Verification items for the finished model (mm, model axes). Face numbers are marked on the shaded views. A direction names the side the tool comes from. Coordinates: 2 decimals unless noted, no trailing zeros. Write each loop counter-clockwise with the first axis right and the second up, starting at its lowest first coordinate (ties: lowest second). Pieces come first, ordered by that corner, then holes. Notation, with made-up numbers: (27, -22.5) -> (52, -22.5) arc R19 cw to (52, 11.5) -> close; hole circle Ø11 at (-7.75, 77.25). An arc over 180 degrees is marked (long way). Use a Markdown table: item, result. Add a question column.
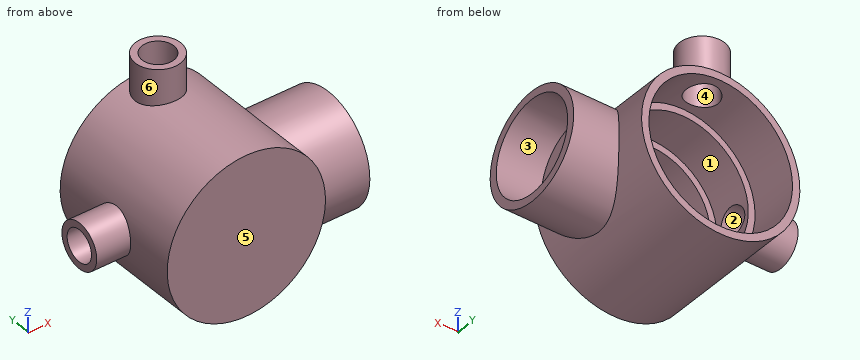
from build123d import *

# Parameters (mm, degrees)
SKETCH1_R                  = 35
BASE_DEPTH                 = 4
SKETCH2_R                  = 7.5
CENTERING_BOSS_DEPTH       = 2
SKETCH3_R                  = 35
SKETCH3_R_2                = 25.75
INLET_TIER_DEPTH           = 18
SKETCH4_R                  = 35
SKETCH4_R_2                = 28.75
PATIENT_TIER_DEPTH         = 18
SKETCH5_R                  = 35
SKETCH5_R_2                = 31.75
OUTLET_TIER_DEPTH          = 21.5
INLET_REACH                = 116.487
INLET_END_RADIUS           = 35
SKETCH7_R                  = 24
SKETCH10_R                 = 20.5
INLET_ID_DEPTH             = 20
INLET_PASS_THRU_REACH      = 101.535
INLET_PASS_THRU_END_RADIUS = 25.75
SKETCH11_R                 = 6
BOSS_EXTRUDE8_REACH        = 128.619
BOSS_EXTRUDE8_END_RADIUS   = 35
SKETCH12_R                 = 10
CUT_EXTRUDE3_REACH         = 128.619
CUT_EXTRUDE3_END_RADIUS    = 28.75
SKETCH13_R                 = 7
BOSS_EXTRUDE9_REACH        = 120.458
BOSS_EXTRUDE9_END_RADIUS   = 35
SKETCH14_R                 = 10
CUT_EXTRUDE4_REACH         = 120.458
CUT_EXTRUDE4_END_RADIUS    = 31.75
SKETCH15_R                 = 7


with BuildPart() as part:
    # Sketch1 → Base (new body)
    with BuildSketch(Plane(origin=(0, 0, 0), x_dir=(1, 0, 0), z_dir=(0, 1, 0))):
        with Locations(Location((0, 0, 0), (0, 0, 270))):
            Circle(SKETCH1_R)
    extrude(amount=BASE_DEPTH)

    # Sketch2 → Centering boss (add)
    with BuildSketch(Plane(origin=(0, 4, 0), x_dir=(1, 0, 0), z_dir=(0, 1, 0))):
        with Locations(Location((0, 0, 0), (0, 0, 270))):
            Circle(SKETCH2_R)
    extrude(amount=CENTERING_BOSS_DEPTH)

    # Sketch3 → Inlet tier (add)
    with BuildSketch(Plane(origin=(0, 4, 0), x_dir=(1, 0, 0), z_dir=(0, 1, 0))):
        with Locations(Location((0, 0, 0), (0, 0, 270))):
            Circle(SKETCH3_R)
        with Locations(Location((0, 0, 0), (0, 0, 270))):
            Circle(SKETCH3_R_2, mode=Mode.SUBTRACT)
    extrude(amount=INLET_TIER_DEPTH)

    # Sketch4 → Patient tier (add)
    with BuildSketch(Plane(origin=(0, 22, 0), x_dir=(1, 0, 0), z_dir=(0, 1, 0))):
        with Locations(Location((0, 0, 0), (0, 0, 270))):
            Circle(SKETCH4_R)
        with Locations(Location((0, 0, 0), (0, 0, 270))):
            Circle(SKETCH4_R_2, mode=Mode.SUBTRACT)
    extrude(amount=PATIENT_TIER_DEPTH)

    # Sketch5 → Outlet tier (add)
    with BuildSketch(Plane(origin=(0, 40, 0), x_dir=(1, 0, 0), z_dir=(0, 1, 0))):
        with Locations(Location((0, 0, 0), (0, 0, 270))):
            Circle(SKETCH5_R)
        with Locations(Location((0, 0, 0), (0, 0, 270))):
            Circle(SKETCH5_R_2, mode=Mode.SUBTRACT)
    extrude(amount=OUTLET_TIER_DEPTH)

    # Inlet: up to this cylinder (the profile starts outside it)
    inlet_end = Plane(origin=(0, 24.5, 0), z_dir=(0, -1, 0)) * Cylinder(INLET_END_RADIUS, 303.974, mode=Mode.PRIVATE)
    # Sketch7 → Inlet (add, up to the surface)
    with BuildSketch(Plane(origin=(55, 0, 0), x_dir=(0, 0, -1), z_dir=(1, 0, 0)), mode=Mode.PRIVATE) as inlet_sk1:
        with Locations((0, 24.5)):
            Circle(SKETCH7_R)
    inlet_tool1 = extrude(inlet_sk1.sketch, amount=-INLET_REACH, mode=Mode.PRIVATE) - inlet_end
    add(inlet_tool1.solids().sort_by_distance((55, 24.5, 0))[0])

    # Sketch10 → Inlet ID (cut)
    with BuildSketch(Plane(origin=(55, 0, 0), x_dir=(0, 0, -1), z_dir=(1, 0, 0))):
        with Locations((0, 24.5)):
            Circle(SKETCH10_R)
    extrude(amount=-INLET_ID_DEPTH, mode=Mode.SUBTRACT)

    # Inlet pass thru: up to this cylinder (the profile starts outside it)
    inlet_pass_thru_end = Plane(origin=(0, 14, 0), z_dir=(0, -1, 0)) * Cylinder(INLET_PASS_THRU_END_RADIUS, 255.57, mode=Mode.PRIVATE)
    # Sketch11 → Inlet pass thru (cut, up to the surface)
    with BuildSketch(Plane(origin=(35, 0, 0), x_dir=(0, 0, -1), z_dir=(1, 0, 0)), mode=Mode.PRIVATE) as inlet_pass_thru_sk1:
        with Locations((0, 14)):
            Circle(SKETCH11_R)
    inlet_pass_thru_tool1 = extrude(inlet_pass_thru_sk1.sketch, amount=-INLET_PASS_THRU_REACH, mode=Mode.PRIVATE) - inlet_pass_thru_end
    add(inlet_pass_thru_tool1.solids().sort_by_distance((35, 14, 0))[0], mode=Mode.SUBTRACT)

    # Boss-Extrude8: up to this cylinder (the profile starts outside it)
    boss_extrude8_end = Plane(origin=(0, 31, 0), z_dir=(0, -1, 0)) * Cylinder(BOSS_EXTRUDE8_END_RADIUS, 328.238, mode=Mode.PRIVATE)
    # Sketch12 → Boss-Extrude8 (add, up to the surface)
    with BuildSketch(Plane(origin=(-50, 0, 0), x_dir=(0, 0, -1), z_dir=(1, 0, 0)), mode=Mode.PRIVATE) as boss_extrude8_sk1:
        with Locations(Location((0, 31, 0), (0, 0, 180))):
            Circle(SKETCH12_R)
    boss_extrude8_tool1 = extrude(boss_extrude8_sk1.sketch, amount=BOSS_EXTRUDE8_REACH, mode=Mode.PRIVATE) - boss_extrude8_end
    add(boss_extrude8_tool1.solids().sort_by_distance((-50, 31, 0))[0])

    # Cut-Extrude3: up to this cylinder (the profile starts outside it)
    cut_extrude3_end = Plane(origin=(0, 31, 0), z_dir=(0, -1, 0)) * Cylinder(CUT_EXTRUDE3_END_RADIUS, 315.738, mode=Mode.PRIVATE)
    # Sketch13 → Cut-Extrude3 (cut, up to the surface)
    with BuildSketch(Plane.ZY.offset(50), mode=Mode.PRIVATE) as cut_extrude3_sk1:
        with Locations((0, 31)):
            Circle(SKETCH13_R)
    cut_extrude3_tool1 = extrude(cut_extrude3_sk1.sketch, amount=-CUT_EXTRUDE3_REACH, mode=Mode.PRIVATE) - cut_extrude3_end
    add(cut_extrude3_tool1.solids().sort_by_distance((-50, 31, 0))[0], mode=Mode.SUBTRACT)

    # Boss-Extrude9: up to this cylinder (the profile starts outside it)
    boss_extrude9_end = Plane(origin=(0, 50.75, 0), z_dir=(0, -1, 0)) * Cylinder(BOSS_EXTRUDE9_END_RADIUS, 311.916, mode=Mode.PRIVATE)
    # Sketch14 → Boss-Extrude9 (add, up to the surface)
    with BuildSketch(Plane.XY.offset(50), mode=Mode.PRIVATE) as boss_extrude9_sk1:
        with Locations((0, 50.75)):
            Circle(SKETCH14_R)
    boss_extrude9_tool1 = extrude(boss_extrude9_sk1.sketch, amount=-BOSS_EXTRUDE9_REACH, mode=Mode.PRIVATE) - boss_extrude9_end
    add(boss_extrude9_tool1.solids().sort_by_distance((0, 50.75, 50))[0])

    # Cut-Extrude4: up to this cylinder (the profile starts outside it)
    cut_extrude4_end = Plane(origin=(0, 50.75, 0), z_dir=(0, -1, 0)) * Cylinder(CUT_EXTRUDE4_END_RADIUS, 305.416, mode=Mode.PRIVATE)
    # Sketch15 → Cut-Extrude4 (cut, up to the surface)
    with BuildSketch(Plane.XY.offset(50), mode=Mode.PRIVATE) as cut_extrude4_sk1:
        with Locations((0, 50.75)):
            Circle(SKETCH15_R)
    cut_extrude4_tool1 = extrude(cut_extrude4_sk1.sketch, amount=-CUT_EXTRUDE4_REACH, mode=Mode.PRIVATE) - cut_extrude4_end
    add(cut_extrude4_tool1.solids().sort_by_distance((0, 50.75, 50))[0], mode=Mode.SUBTRACT)


solid = part.part
1) Release check for a two-part mould opening along X. For the marked faces 4, 5 and 6 record: released by +X, released by -X, zero draft, split by the parting line, or undercut.
2) Thickness scan on L1, parallel to Y at x = 0, z = 38.75; L2, parallel to Y at x = 40, z = 0; L3, parallel to Z at x = -41, y = 31. Record the ranges inside material, lowest first.
3) Cross-section at A-A on x = 0. Record the boundary of the cut face in (y, z), then the cut area to 3 significant figures.
4) Cross-section at D-D on y = 14. Record the boundary of the cut face in (x, z).
5) Cross-section at B-B on z = -18. Record the boundary of the cut face in (x, y).
6) Cross-section at C-C on x = -20. Record the boundary of the cut face in (y, z), then the cut area to 3 significant figures.
7) Set-up check for the marked faces 1, 2 and 3: record each of +Z, -Z, +X, -X, +Y, -Y from which the full face is reachable in a straight line by a thin tool's end or side.
8) Gauge pin test, flat ends, axial feed: pin 1 (19 mm diameter, centred on y = 14, z = 0, fed in from -X); pin 2 (20.5 mm diameter, centred on y = 19, z = 2.5, fed in from +X); pin 3 (1 mm diameter, centred on y = 13.5, z = -21.5, fed in from -X); pin 4 (2 mm diameter, centred on y = 10.5, z = -7.5, fed in from -X). Record the tip position at first contact, or that the pin passes through.
Returned:
| question | item | result |
|---|---|---|
| 1 | face 4 | undercut |
| 1 | face 5 | zero draft |
| 1 | face 6 | split by the parting line |
| 2 | L1 | y = 40.75 to 43.75, 57.75 to 60.75 |
| 2 | L2 | y = 0.5 to 4, 45 to 48.5 |
| 2 | L3 | z = -10 to -7, 7 to 10 |
| 3 | outline | (0, -35) -> (61.5, -35) -> (61.5, -31.75) -> (40, -31.75) -> (40, -28.75) -> (22, -28.75) -> (22, -25.75) -> (4, -25.75) -> (4, -7.5) -> (6, -7.5) -> (6, 7.5) -> (4, 7.5) -> (4, 25.75) -> (22, 25.75) -> (22, 28.75) -> (40, 28.75) -> (40, 31.75) -> (43.75, 31.75) -> (43.75, 50) -> (40.75, 50) -> (40.75, 35) -> (0, 35) -> close; (57.75, 31.75) -> (61.5, 31.75) -> (61.5, 35) -> (60.75, 35) -> (60.75, 50) -> (57.75, 50) -> close |
| 3 | area | 1,050 mm² |
| 4 | outline | (25.04, -6) arc R25.75 cw (long way) to (25.04, 6) -> (35, 6) -> (35, 17.61) -> (55, 17.61) -> (55, 21.58) -> (27.55, 21.58) arc R35 ccw (long way) to (27.55, -21.58) -> (55, -21.58) -> (55, -17.61) -> (35, -17.61) -> (35, -6) -> close |
| 5 | outline | (-30.02, 0) -> (30.02, 0) -> (30.02, 8.63) -> (55, 8.63) -> (55, 14.69) -> (35, 14.69) -> (35, 34.31) -> (55, 34.31) -> (55, 40.37) -> (30.02, 40.37) -> (30.02, 61.5) -> (26.15, 61.5) -> (26.15, 40) -> (22.42, 40) -> (22.42, 22) -> (18.41, 22) -> (18.41, 4) -> (-18.41, 4) -> (-18.41, 22) -> (-22.42, 22) -> (-22.42, 40) -> (-26.15, 40) -> (-26.15, 61.5) -> (-30.02, 61.5) -> close |
| 6 | outline | (0, -28.72) -> (61.5, -28.72) -> (61.5, -24.66) -> (40, -24.66) -> (40, -20.65) -> (22, -20.65) -> (22, -16.22) -> (4, -16.22) -> (4, 16.22) -> (22, 16.22) -> (22, 20.65) -> (40, 20.65) -> (40, 24.66) -> (61.5, 24.66) -> (61.5, 28.72) -> (0, 28.72) -> close |
| 6 | area | 1,150 mm² |
| 7 | face 1 | +Y |
| 7 | face 2 | -X |
| 7 | face 3 | +X |
| 8 | pin 1 | stops at x = -50 |
| 8 | pin 2 | stops at x = 35 |
| 8 | pin 3 | stops at x = -28 |
| 8 | pin 4 | stops at x = -34.39 |
